from build123d import *

# Parameters (mm, degrees)
SKETCH_1_W          = 76
SKETCH_1_H          = 60
EXTRUDE_1_DEPTH     = 0.13
SKETCH_2_W          = 30
SKETCH_2_H          = 10
CUT_EXTRUDE_1_DEPTH = 49.41504828
CUT_EXTRUDE_2_DEPTH = 49.41504828


with BuildPart() as part:
    # 草圖1 → 填料-伸長1 (new body)
    with BuildSketch(Plane.XY):
        Rectangle(SKETCH_1_W, SKETCH_1_H)
    extrude(amount=EXTRUDE_1_DEPTH)

    # 草圖2 → 除料-伸長1 (cut, through all)
    with BuildSketch(Plane.XY.offset(0.13)):
        with Locations((-23, 25)):
            Rectangle(SKETCH_2_W, SKETCH_2_H)
        with Locations((23, 25)):
            Rectangle(SKETCH_2_W, SKETCH_2_H)
        with Locations((23, -25)):
            Rectangle(SKETCH_2_W, SKETCH_2_H)
        with Locations((-23, -25)):
            Rectangle(SKETCH_2_W, SKETCH_2_H)
    extrude(amount=-CUT_EXTRUDE_1_DEPTH, mode=Mode.SUBTRACT)

    # 草圖3 → 除料-伸長2 (cut, through all)
    with BuildSketch(Plane.XY.offset(0.13)):
        with BuildLine():
            Line((-8, 19.4), (-29.9, 19.4))
            ThreePointArc((-29.9, 19.4), (-33.435533906, 17.935533906), (-34.9, 14.4))
            Line((-34.9, 14.4), (-34.9, -14.4))
            ThreePointArc((-34.9, -14.4), (-33.435533906, -17.935533906), (-29.9, -19.4))
            Line((-29.9, -19.4), (-8, -19.4))
            Line((-8, -19.4), (-8, -20))
            Line((-8, -20), (-38, -20))
            Line((-38, -20), (-38, 20))
            Line((-38, 20), (-8, 20))
            Line((-8, 20), (-8, 19.4))
        make_face()
        with BuildLine():
            Line((8, -20), (8, -19.4))
            Line((8, -19.4), (29.9, -19.4))
            ThreePointArc((29.9, -19.4), (33.435533906, -17.935533906), (34.9, -14.4))
            Line((34.9, -14.4), (34.9, 14.4))
            ThreePointArc((34.9, 14.4), (33.435533906, 17.935533906), (29.9, 19.4))
            Line((29.9, 19.4), (8, 19.4))
            Line((8, 19.4), (8, 20))
            Line((8, 20), (38, 20))
            Line((38, 20), (38, -20))
            Line((38, -20), (8, -20))
        make_face()
    extrude(amount=-CUT_EXTRUDE_2_DEPTH, mode=Mode.SUBTRACT)


solid = part.part
Here's how the part is built. I have some questions about the finished solid (model axes, mm). Round coordinates to 2 decimals unless told otherwise and drop trailing zeros. Loops run counter-clockwise (first coordinate to the right, second up) from the corner with the lowest first, then second, coordinate; pieces in that order, holes last. Notation, with made-up numbers: (2, 38) -> (36, 38) arc R28 ccw to (36, 74) -> close; hole circle Ø5 at (35.25, 80). An arc over 180 degrees is marked (long way). Write each question's results on one line, items separated by ' | '.
(1) If we section it at C-C, the plane y = -17.5: List the corners of the cut face in (x, z) for me.
Worked answers:
outline: (-33.82, 0) -> (33.82, 0) -> (33.82, 0.13) -> (-33.82, 0.13) -> close
(2) If we section it at A-A, the plane z = 0.05: List the corners of the cut face in (x, y) for me.
Worked answers:
outline: (-34.9, -14.4) arc R5 ccw to (-29.9, -19.4) -> (-8, -19.4) -> (-8, -30) -> (8, -30) -> (8, -19.4) -> (29.9, -19.4) arc R5 ccw to (34.9, -14.4) -> (34.9, 14.4) arc R5 ccw to (29.9, 19.4) -> (8, 19.4) -> (8, 30) -> (-8, 30) -> (-8, 19.4) -> (-29.9, 19.4) arc R5 ccw to (-34.9, 14.4) -> close
(3) If we section it at B-B, the plane x = 27.5: List the corners of the cut face in (y, z) for me.
Worked answers:
outline: (-19.4, 0) -> (19.4, 0) -> (19.4, 0.13) -> (-19.4, 0.13) -> close
(4) If I drill on L1, parallel to X at y = 23.5, z = 0.05; L2, parallel to Y at x = -11, z = 0.05, over which ranges is the centre line in solid material (lowest first)?
Worked answers:
L1: -8 to 8 | L2: -19.4 to 19.4
